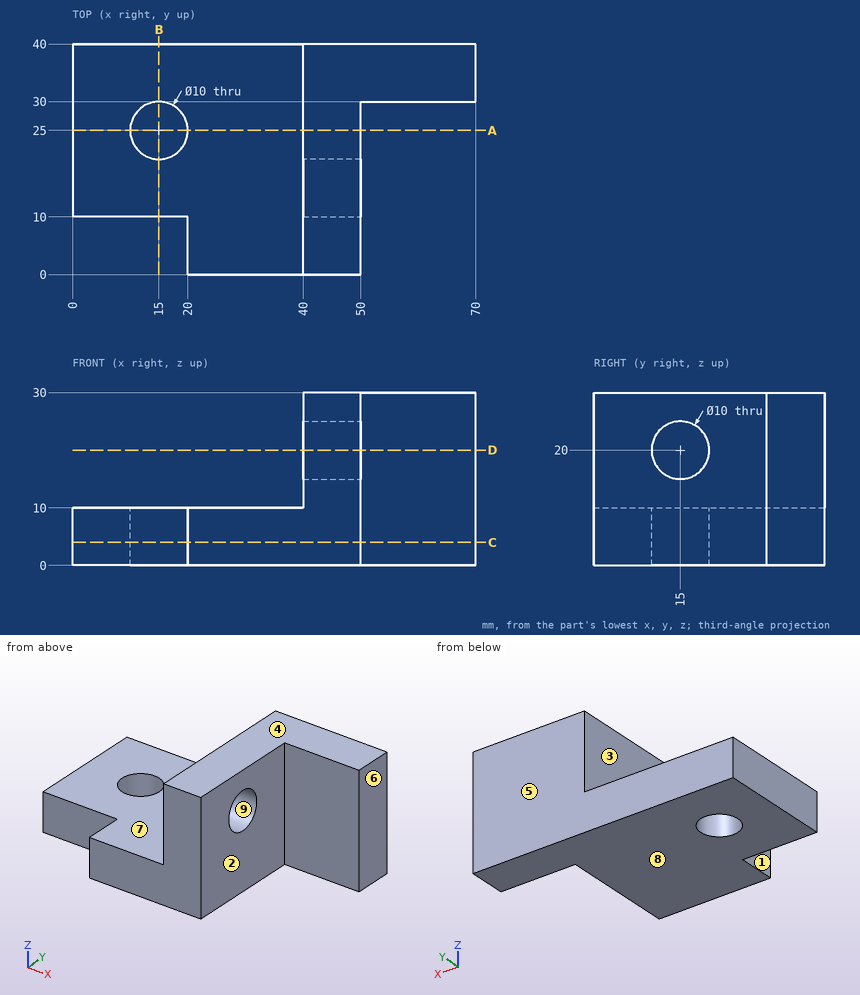
Source: three-view drawing plus pictorial views. Frame: mm from the lowest corner of the part. A direction names the side the tool comes from. Give positions to 0.01 mm unless a question says otherwise; leave off trailing zeros. Write each loop counter-clockwise with the first axis right and the second up, starting at its lowest first coordinate (ties: lowest second). Pieces come first, ordered by that corner, then holes. Notation, with made-up numbers: (41.25, 57) - (77.25, 57) arc R36 ccw to (77.25, 93) - close; hole circle Ø2 at (-31, 33). An arc over 180 degrees is marked (long way). Write item = value, one per line. Start each with the question number.
1. Section query C-C, the plane z = 4. Output: boundary loops of the cut face in (x, y), then the cut area to 3 significant figures.
2. Access query for the marked faces 1, 2, 3, 4 and 5. Directions: +Z, -Z, +X, -X, +Y, -Y. A direction counts if a zero-diameter tool reaches every point of the face in a straight line with its end or side. Return the directions, or none.
3. Section query A-A, the plane y = 25. Output: boundary loops of the cut face in (x, z).
4. First-contact query: pin 1 Ø9 at (y, z) = (8, 21.5) entering from +X; pin 2 Ø3 at (y, z) = (9, 16.5) entering from -X; pin 3 Ø6 at (y, z) = (15, 20) entering from -X; pin 4 Ø3 at (y, z) = (6.5, 4.5) entering from -X. Flat tips, straight axial feed; report the tip coordinate or a pass-through.
5. Mould query, pull axis Z, two halves, no side actions, for the marked faces 6, 7, 8 and 9. Classes: released by +Z, released by -Z, zero draft, split by the parting line, or undercut.
6. Section query D-D, the plane z = 20. Output: boundary loops of the cut face in (x, y).
7. Section query B-B, the plane x = 15. Output: boundary loops of the cut face in (y, z), then the cut area to 3 significant figures.
8. Ray query, L1, parallel to Z at x = 44, y = 15; L2, parallel to X at y = 35.5, z = 21.75; L3, parallel to X at y = 7.5, z = 15.5. Return the intervals inside material, ascending.
Check sheet entries:
q1.outline = (0, 10) - (20, 10) - (20, 0) - (50, 0) - (50, 30) - (70, 30) - (70, 40) - (0, 40) - close; hole circle Ø10 at (15, 25)
q1.area = 1,920 mm2
q2.face_1 = +Z, -Z, -X, -Y
q2.face_2 = +Z, -Z, +X, -Y
q2.face_3 = +Z, -X, +Y, -Y
q2.face_4 = +Z, +X, -X, +Y, -Y
q2.face_5 = +Z, -Z, +X, -X, +Y
q3.outline = (0, 0) - (10, 0) - (10, 10) - (0, 10) - close; (20, 0) - (50, 0) - (50, 30) - (40, 30) - (40, 10) - (20, 10) - close
q4.pin_1 = 50
q4.pin_2 = 40
q4.pin_3 = through
q4.pin_4 = 20
q5.face_6 = zero draft
q5.face_7 = released by +Z
q5.face_8 = released by -Z
q5.face_9 = undercut
q6.outline = (40, 0) - (50, 0) - (50, 10) - (40, 10) - close; (40, 20) - (50, 20) - (50, 30) - (70, 30) - (70, 40) - (40, 40) - close
q7.outline = (10, 0) - (20, 0) - (20, 10) - (10, 10) - close; (30, 0) - (40, 0) - (40, 10) - (30, 10) - close
q7.area = 200 mm2
q8.L1 = 0 to 15, 25 to 30
q8.L2 = 40 to 70
q8.L3 = 40 to 50
